The model under review builds one solid part; all positions refer to its coordinate system, in mm. A direction names the side the tool comes from. Round coordinates to 2 decimals unless told otherwise and drop trailing zeros. Write each loop counter-clockwise with the first axis right and the second up, starting at its lowest first coordinate (ties: lowest second). Pieces come first, ordered by that corner, then holes. Notation, with made-up numbers: (11.5, -22) -> (15.5, -22) arc R13 ccw to (15.5, -18) -> close; hole circle Ø3 at (7.25, 58). An arc over 180 degrees is marked (long way). Use CSV: the item, a comma, the result in double quotes. Start each with the question number.
1) For pin 1 Ø1 at (x, y) = (-11.5, 4) entering from +Z, flat-tipped, find the tip position at first contact; note if it passes through.
2) Machinability: for faces 1 (the face through (-1, 0, 0)), 2 (the face through (-1, -19, 27)), 3 (the face through (-49, 0, 11)), which of the approach directions +Z, -Z, +X, -X, +Y, -Y give a long, thin tool a straight path to every point of the face, cutting with its end or side? Answer none if there is none.
3) Mouldability with a two-part tool opening along Y and no side actions: class faces 4 (the face through (-1, -20, 16)), 5 (the face through (-0.2, 19.4, 32)), 6 (the face through (-1, 19, 11)), 7 (the face through (-1, 20, 16)) as released by +Y, released by -Y, zero draft, split by the parting line, or undercut.
4) Take a section at C-C, the plane z = 23. Give the boundary of the cut face in (x, y), then the cut area to 3 significant figures.
5) Wall thickness on probe 1 along Z at (x, y) = (5.5, 3.5); probe 2 along Y at (x, z) = (-12, 7); probe 3 along X at (y, z) = (-14.5, 22.5): over which ranges is each line inside the solid? List them lowest first. Write a range as [from, to].
6) Take a section at B-B, the plane y = 17.5. Give the boundary of the cut face in (x, z).
7) Take a section at A-A, the plane x = -13. Give the boundary of the cut face in (y, z), then the cut area to 3 significant figures.
from build123d import *

# Parameters (mm, degrees)
F0_W     = 100
F0_H     = 40
F1_DEPTH = 32
F2_T     = -1
F3_W     = 38
F3_H     = 0.2
F4_DEPTH = 98


with BuildPart() as f1:
    # F0 (on Top) → F1 (new body)
    with BuildSketch(Plane.XY):
        Rectangle(F0_W, F0_H)
    extrude(amount=F1_DEPTH)

    # F2
    f2_openings = [f1.faces().sort_by_distance(p)[0] for p in [
        (0, 0, 32),
    ]]
    offset(amount=F2_T, openings=f2_openings)

    # F3 (on face) → F4 (join, through all)
    with BuildSketch(Plane.YZ.offset(-49)):
        with Locations((0, 21.1)):
            Rectangle(F3_W, F3_H)
    extrude(amount=F4_DEPTH)


solid = f1.part
Values found:
1,pin 1,"z = 21.2"
2,face 1,"-Z, +X, -X, +Y, -Y"
2,face 2,"+Z"
2,face 3,"none"
3,face 4,"released by -Y"
3,face 5,"zero draft"
3,face 6,"undercut"
3,face 7,"released by +Y"
4,outline,"(-50, -20) -> (50, -20) -> (50, 20) -> (-50, 20) -> close; hole (-49, -19) -> (49, -19) -> (49, 19) -> (-49, 19) -> close"
4,area,"276 mm²"
5,probe 1,"[0, 1], [21, 21.2]"
5,probe 2,"[-20, -19], [19, 20]"
5,probe 3,"[-50, -49], [49, 50]"
6,outline,"(-50, 0) -> (50, 0) -> (50, 32) -> (49, 32) -> (49, 21.2) -> (-49, 21.2) -> (-49, 32) -> (-50, 32) -> close; hole (-49, 1) -> (49, 1) -> (49, 21) -> (-49, 21) -> close"
7,outline,"(-20, 0) -> (20, 0) -> (20, 32) -> (19, 32) -> (19, 21.2) -> (-19, 21.2) -> (-19, 32) -> (-20, 32) -> close; hole (-19, 1) -> (19, 1) -> (19, 21) -> (-19, 21) -> close"
7,area,"110 mm²"
